Part model, mm, in its own coordinate system. A direction names the side the tool comes from. Give positions to 0.01 mm unless a question says otherwise; leave off trailing zeros. Order: outer loops, then holes, each group sorted by start corner. A loop starts at its lowest first (then second) coordinate and runs counter-clockwise, first axis right, second up. Notation, with made-up numbers: (39.25, -14.75) - (51.25, -14.75) arc R29 cw to (51.25, 8.25) - close; hole circle Ø8 at (26.25, 6). An arc over 180 degrees is marked (long way). One line per item, written item: value.
Autodesk Fusion 360 part; units mm, degrees
sketch "Sketch1" plane through (0, 0, 0) normal (1, 0, 0) x (0, 1, 0)
  line L0 (-60.2, 30) -> (-60.2, 0)
  line L1 (-60.2, 0) -> (-37.3, 0)
  line L2 (-37.3, 0) -> (-37.3, 10)
  line L3 (-37.3, 10) -> (-32.5, 10)
  line L4 (-32.5, 10) -> (-32.5, 0)
  line L5 (-32.5, 0) -> (32.5, 0)
  line L6 (32.5, 0) -> (32.5, 10)
  line L7 (32.5, 10) -> (37.3, 10)
  line L8 (37.3, 10) -> (37.3, 0)
  line L9 (37.3, 0) -> (60.2, 0)
  line L10 (60.2, 0) -> (60.2, 30)
  line L11 (60.2, 30) -> (55.2, 30)
  line L12 (55.2, 30) -> (55.2, 15)
  line L13 (55.2, 15) -> (50.4, 15)
  line L14 (50.4, 15) -> (50.4, 30)
  line L15 (50.4, 30) -> (-50.4, 30)
  line L16 (-50.4, 30) -> (-50.4, 15)
  line L17 (-50.4, 15) -> (-55.2, 15)
  line L18 (-55.2, 15) -> (-55.2, 30)
  line L19 (-55.2, 30) -> (-60.2, 30)
  line L20 (-55.2, 30) -> (-50.4, 30) construction
  line L21 (50.4, 30) -> (55.2, 30) construction
  line L22 (37.3, 0) -> (32.5, 0) construction
  line L23 (-32.5, 0) -> (-37.3, 0) construction
  line L24 (-50.4, 15) -> (50.4, 15) construction
  line L25 (0, 0) -> (0, 15) construction
  line L26 (0, 15) -> (0, 30) construction
  circle A0 centre (0, 15) radius 1.5
  circle A1 centre (-45.4, 15) radius 1.5
  circle A2 centre (45.4, 15) radius 1.5
  line L27 (-32.5, 10) -> (32.5, 10) construction
  point P0 (0, 15)
  point P1 (0, 15)
  point P2 (0, 30)
  dimension "d1" = 4.8
  dimension "d2" = 4.8
  dimension "d3" = 4.8
  dimension "d4" = 4.8
  dimension "d7" = 15
  dimension "d9" = 30
  dimension "d10" = 65
  dimension "d11" = 120.4
  dimension "d12" = 100.8
  dimension "d13" = 5
  dimension "d14" = 3
  dimension "d15" = 3
  dimension "d16" = 5
  dimension "d17" = 3
  dimension "d18" = 5
  dimension "d21" = 10
extrude "Extrude1" add sketch "Sketch1" along normal blind 4.8
1) Which spindle directions (+Z, -Z, +X, -X, +Y, -Y) get a long thin tool onto all of the face, cutting with end or side? Do faces 1 (the flat face through (2, 50.4, 22)), 2 (the flat face through (2, 37.3, 5)), 3 (the flat face through (0, -1, 12)). Say none if no direction does.
Outcome:
face 1: +Z, +X, -X
face 2: -Z, +X, -X
face 3: +Z, -Z, -X, +Y, -Y
2) Cut at C-C, the plane z = 27. Give the cut face in (x, y).
Outcome:
outline: (0, -60.2) - (4.8, -60.2) - (4.8, -55.2) - (0, -55.2) - close; (0, -50.4) - (4.8, -50.4) - (4.8, 50.4) - (0, 50.4) - close; (0, 55.2) - (4.8, 55.2) - (4.8, 60.2) - (0, 60.2) - close
3) Cut at A-A, the plane y = 0. Give the cut face in (x, z).
Outcome:
outline: (0, 0) - (4.8, 0) - (4.8, 13.5) - (0, 13.5) - close; (0, 16.5) - (4.8, 16.5) - (4.8, 30) - (0, 30) - close
4) Drill centre lines: line 1 along Y through (x, z) = (0.3, 28.75); line 2 along Y through (x, z) = (4.6, 8.75); line 3 along Z through (x, y) = (2.2, 0). Where is each one in solid material? Low to high. Write a range as from..to.
Outcome:
line 1: y = -60.2..-55.2, -50.4..50.4, 55.2..60.2
line 2: y = -60.2..-37.3, -32.5..32.5, 37.3..60.2
line 3: z = 0..13.5, 16.5..30
5) Cut at B-B, the plane x = 1.2. Give the cut face in (y, z), then the cut area to 3 significant figures.
Outcome:
outline: (-60.2, 0) - (-37.3, 0) - (-37.3, 10) - (-32.5, 10) - (-32.5, 0) - (32.5, 0) - (32.5, 10) - (37.3, 10) - (37.3, 0) - (60.2, 0) - (60.2, 30) - (55.2, 30) - (55.2, 15) - (50.4, 15) - (50.4, 30) - (-50.4, 30) - (-50.4, 15) - (-55.2, 15) - (-55.2, 30) - (-60.2, 30) - close; hole circle Ø3 at (-45.4, 15); hole circle Ø3 at (0, 15); hole circle Ø3 at (45.4, 15)
area: 3,350 mm^2
6) Mould opens along Z. For faces 4 (the cylindrical face through (2.4, -46.6, 15.9)), 5 (the flat face through (2, 32.5, 5)), 6 (the flat face through (2, 1, 30)) say: released by +Z, released by -Z, zero draft, split by the parting line, or undercut.
Outcome:
face 4: undercut
face 5: zero draft
face 6: released by +Z
